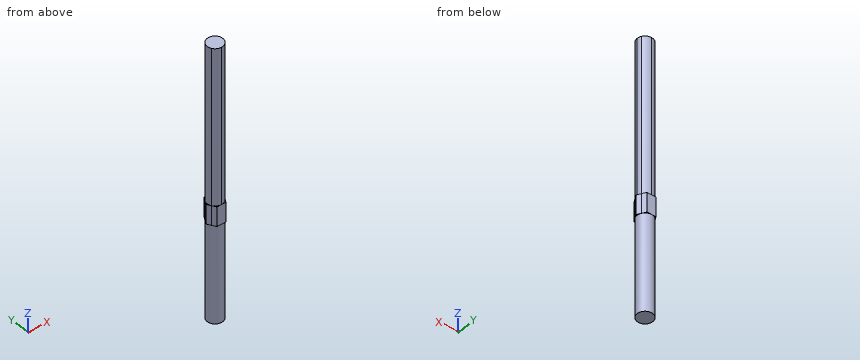
```python
from build123d import *

# Parameters (mm, degrees)
F0_R     = 2
F1_DEPTH = 25
F3_DEPTH = 5
F5_DEPTH = 40


with BuildPart() as f1:
    # F0 (on Top) → F1 (new body)
    with BuildSketch(Plane.XY):
        Circle(F0_R)
    extrude(amount=F1_DEPTH)

    # F2 (on face) → F3 (join)
    with BuildSketch(Plane.XY.offset(25)):
        with BuildLine():
            Line((0, 2), (-1.1547005384, 2))
            Line((-1.1547005384, 2), (-1.7320507826, 1.0000000433))
            ThreePointArc((-1.7320507826, 1.0000000433), (-0.9999999783, 1.7320508201), (0, 2))
        make_face()
        with BuildLine():
            ThreePointArc((-1.7320507826, -1.0000000433), (-2, 0), (-1.7320507826, 1.0000000433))
            Line((-1.7320507826, 1.0000000433), (-2.3094010768, 0))
            Line((-2.3094010768, 0), (-1.7320507826, -1.0000000433))
        make_face()
        with BuildLine():
            ThreePointArc((0, -2), (-0.9999999783, -1.7320508201), (-1.7320507826, -1.0000000433))
            Line((-1.7320507826, -1.0000000433), (-1.1547005384, -2))
            Line((-1.1547005384, -2), (0, -2))
        make_face()
        with BuildLine():
            ThreePointArc((1.7320507983, -1.0000000161), (0.999999992, -1.7320508122), (0, -2))
            Line((0, -2), (1.1547005384, -2))
            Line((1.1547005384, -2), (1.7320507983, -1.0000000161))
        make_face()
        with BuildLine():
            Line((2.3094010768, 0), (1.7320507826, 1.0000000433))
            ThreePointArc((1.7320507826, 1.0000000433), (1.9318516461, 0.5176381144), (2, 0))
            ThreePointArc((2, 0), (1.9318516502, -0.5176380992), (1.7320507983, -1.0000000161))
            Line((1.7320507983, -1.0000000161), (2.3094010768, 0))
        make_face()
        with BuildLine():
            Line((1.1547005384, 2), (0, 2))
            ThreePointArc((0, 2), (0.9999999783, 1.7320508201), (1.7320507826, 1.0000000433))
            Line((1.7320507826, 1.0000000433), (1.1547005384, 2))
        make_face()
        with BuildLine():
            ThreePointArc((1.7320507826, 1.0000000433), (0.9999999783, 1.7320508201), (0, 2))
            ThreePointArc((0, 2), (-0.9999999783, 1.7320508201), (-1.7320507826, 1.0000000433))
            ThreePointArc((-1.7320507826, 1.0000000433), (-2, 0), (-1.7320507826, -1.0000000433))
            ThreePointArc((-1.7320507826, -1.0000000433), (-0.9999999783, -1.7320508201), (0, -2))
            ThreePointArc((0, -2), (0.999999992, -1.7320508122), (1.7320507983, -1.0000000161))
            ThreePointArc((1.7320507983, -1.0000000161), (1.9318516502, -0.5176380992), (2, 0))
            ThreePointArc((2, 0), (1.9318516461, 0.5176381144), (1.7320507826, 1.0000000433))
        make_face()
    extrude(amount=F3_DEPTH)

    # F4 (on face) → F5 (join)
    with BuildSketch(Plane.XY.offset(30)):
        with BuildLine():
            ThreePointArc((1.732050814, -0.9999999889), (1.9318516542, -0.517638084), (2, 0))
            ThreePointArc((2, 0), (1.9318516461, 0.5176381144), (1.7320507826, 1.0000000433))
            ThreePointArc((1.7320507826, 1.0000000433), (0.9999999783, 1.7320508201), (0, 2))
            ThreePointArc((0, 2), (-1.0000000056, 1.7320508044), (-1.732050814, 0.9999999889))
            ThreePointArc((-1.732050814, 0.9999999889), (-2, -3.14e-08), (-1.7320507826, -1.0000000433))
            ThreePointArc((-1.7320507826, -1.0000000433), (-0.9999999783, -1.7320508201), (0, -2))
            ThreePointArc((0, -2), (1.0000000056, -1.7320508044), (1.732050814, -0.9999999889))
        make_face()
    extrude(amount=F5_DEPTH)


solid = f1.part
```
Verification items for the finished model (mm, model axes). Coordinates: 2 decimals unless noted, no trailing zeros. Loops run counter-clockwise (first coordinate to the right, second up) from the corner with the lowest first, then second, coordinate; pieces in that order, holes last. Notation, with made-up numbers: (14, 72.25) -> (54, 72.25) arc R22 ccw to (54, 87.25) -> close; hole circle Ø1 at (51, 19.25). An arc over 180 degrees is marked (long way). Answer in a Markdown table with one row per item.
1) Depth check by flat-ended pin: P1, Ø1.5, axis at y = 1, z = 26.5, coming from the +X side. Enter the tip coordinate at first touch or a pass-through.
The answers:
| item | result |
|---|---|
| P1 | stops at x = 2.17 |
2) Section check A-A (z = 47). Record the cut outline in (x, y).
The answers:
| item | result |
|---|---|
| outline | circle Ø4 at (0, 0) |
3) Scan lines: line 1 along Y through (x, z) = (1, 45.5); line 2 along Y through (x, z) = (0.15, 3). Record each from-to range of solid material in increasing order. Write a range as from..to.
The answers:
| item | result |
|---|---|
| line 1 | y = -1.73..1.73 |
| line 2 | y = -1.99..1.99 |
